Design review of the part built by this model. Coordinates are the model's own, in mm. Face numbers are marked on the shaded views. A direction names the side the tool comes from. Give positions to 0.01 mm unless a question says otherwise; leave off trailing zeros. Order: outer loops, then holes, each group sorted by start corner. A loop starts at its lowest first (then second) coordinate and runs counter-clockwise, first axis right, second up. Notation, with made-up numbers: M 31.5,-27 L 69.5,-27 A17 cw 69.5,-2 Z; hole C 31,13.25 d10. An arc over 180 degrees is marked long. Answer as a JSON object with one key per item and string values.
from build123d import *

# Parameters (mm, degrees)
SKETCH1_R           = 20
SKETCH1_R_2         = 3.125
BOSS_EXTRUDE1_DEPTH = 15
SKETCH2_R           = 16.5
SKETCH2_R_2         = 5
CUT_EXTRUDE1_DEPTH  = 5


# Read off the part's stored shape, not the designer's step: Revolve-Thin19
with BuildPart() as part:
    # Sketch1 → Boss-Extrude1 (new body)
    with BuildSketch(Plane.XY):
        Circle(SKETCH1_R)
        Circle(SKETCH1_R_2, mode=Mode.SUBTRACT)
    extrude(amount=BOSS_EXTRUDE1_DEPTH)

    # Sketch2 → Cut-Extrude1 (cut)
    with BuildSketch(Plane.XY.offset(15)):
        Circle(SKETCH2_R)
        Circle(SKETCH2_R_2, mode=Mode.SUBTRACT)
    cut_extrude1 = extrude(amount=-CUT_EXTRUDE1_DEPTH, mode=Mode.SUBTRACT)

    # Mirror1: Cut-Extrude1 across plane
    add(cut_extrude1.mirror(Plane.XY.offset(7.5)), mode=Mode.SUBTRACT)

    # Revolve-Thin19 outline → Revolve-Thin19 (revolve)
    with BuildSketch(Plane.XZ):
        Polygon((10, 1.070581714), (10, 0), (16.5, 0), (16.5, 5), (6.348063393, 5), align=None)
        Polygon((20, 0), (21, 0), (21, 5.392941829), (20, 6.468923892), align=None)
        Polygon((20, 8.634806339), (21, 9.564189861), (21, 15), (20, 15), align=None)
        Polygon((16.5, 10), (16.5, 15), (10, 15), (10, 14.358101386), (5.310761078, 10), align=None)
    revolve(axis=Axis((0, 0, 0), (0, 0, 1)))


solid = part.part
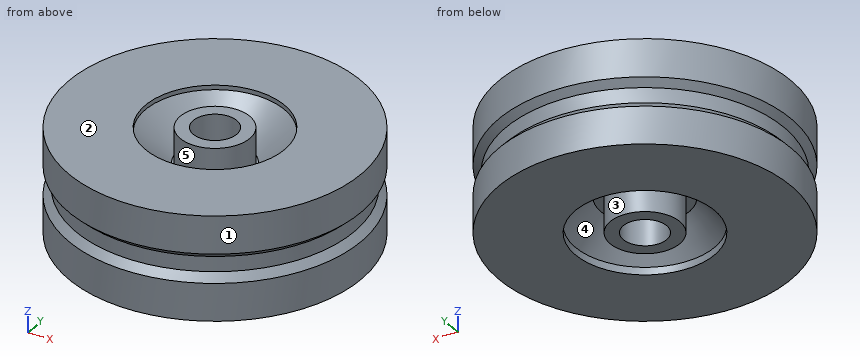
(1) Tool access review of the marked faces 4 and 5: name each direction out of +Z, -Z, +X, -X, +Y, -Y from which nothing blocks a thin tool from reaching the whole face with its end or side.
Checked values:
{"face 4": "-Z", "face 5": "+Z"}
(2) Insertion check: pin 1 (1.5 mm diameter, centred on y = -13, z = 6, fed in from -X); pin 2 (16 mm diameter, centred on x = 0, y = 0, fed in from +Z); pin 3 (6 mm diameter, centred on y = 14.5, z = 9, fed in from -X); pin 4 (6 mm diameter, centred on y = 10, z = 10.5, fed in from -X). Each pin has a flat end and moves straight along its axis. Give the tip position at first contact, or say it passes through.
Checked values:
{"pin 1": "stops at x = -16.83", "pin 2": "stops at z = 15", "pin 3": "stops at x = -17.54", "pin 4": "stops at x = -19.8"}
(3) To check wall thickness, follow L1, parallel to Y at x = 0, z = 14.8 (3 decimals); L2, parallel to X at y = -4, z = 12.5; L3, parallel to Y at x = 0, z = 4.75 (3 decimals). State the ranges of each line that lie inside material, in increasing order. Write a range as from..to.
Checked values:
{"L1": "y = -21..-10, -5..-3.125, 3.125..5, 10..21", "L2": "x = -20.62..-6.93, -3..3, 6.93..20.62", "L3": "y = -21..-6.58, -5..-3.125, 3.125..5, 6.58..21"}
(4) We need section A-A (z = 3). Write out the cut boundary in (x, y) (3 decimals).
Checked values:
{"outline": "C 0,0 d42; C 0,0 d10; hole C 0,0 d16.414; hole C 0,0 d6.25"}
(5) We need section B-B (z = 11.5). Write out the cut boundary in (x, y) (3 decimals).
Checked values:
{"outline": "C 0,0 d42; C 0,0 d10; hole C 0,0 d13.849; hole C 0,0 d6.25"}
(6) Draft analysis for pull direction X (two halves, no side actions). For the marked faces 1, 2 and 3, state which applies: +X half, -X half, draft (parallel to the pull), parting line (faces both ways), or undercut.
Checked values:
{"face 1": "parting line", "face 2": "draft", "face 3": "undercut"}
